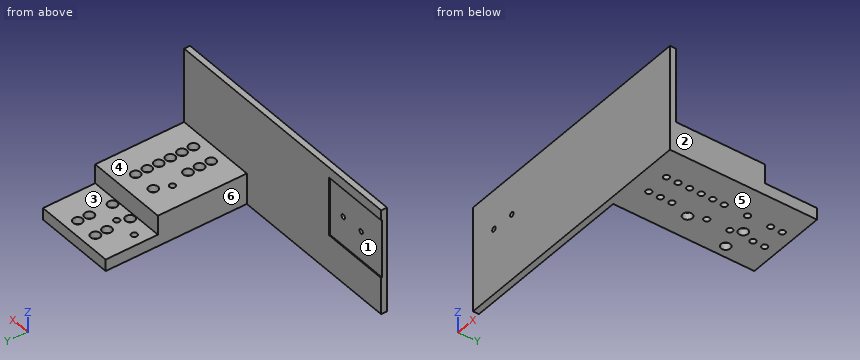
Autodesk Inventor part; units mm, degrees
ref_plane "YZ Plane" through (0, 0, 0) normal (1, 0, 0) x (0, 1, 0)
ref_plane "XZ Plane" through (0, 0, 0) normal (0, 1, 0) x (-1, 0, 0)
ref_plane "XY Plane" through (0, 0, 0) normal (0, 0, 1) x (1, 0, 0)
sketch "Sketch1" plane through (0, 0, 0) normal (0, 0, 1) x (1, 0, 0)
  line L0 (44.45, 76.2) -> (-44.45, 76.2)
  line L1 (-44.45, 76.2) -> (-44.45, -76.2)
  line L2 (-44.45, -76.2) -> (44.45, -76.2)
  line L3 (44.45, -76.2) -> (44.45, 76.2)
  line L4 (44.45, 76.2) -> (-44.45, -76.2) construction
  line L5 (-44.45, 76.2) -> (44.45, -76.2) construction
  point P0 (0, 0)
  dimension "d0" = 152.4
  dimension "d1" = 88.9
extrude "Extrusion1" add sketch "Sketch1" along normal blind 12.7
sketch "Sketch2" plane through (0, 0, 12.7) normal (0, 0, 1) x (1, 0, 0)
  line L0 (-44.45, 76.2) -> (-44.45, -76.2)
  line L1 (44.45, -76.2) -> (44.45, 76.2)
  line L2 (-44.45, -76.2) -> (44.45, -76.2)
  line L3 (44.45, -76.2) -> (44.45, 19.812)
  line L4 (44.45, 19.812) -> (-44.45, 19.812)
  line L5 (-44.45, 19.812) -> (-44.45, -76.2)
  point P0 (0, 0)
  dimension "d4" = 96.012
extrude "Extrusion2" add sketch "Sketch2" along normal blind 20.828
sketch "Sketch3" plane through (0, 0, 0) normal (0, 0, -1) x (-1, 0, 0)
  line L0 (-44.45, -76.2) -> (-44.45, 76.2)
  line L1 (44.45, -76.2) -> (-44.45, -76.2)
  point P0 (0, 0)
  point P1 (19.05, -15.24)
  dimension "d14" = 63.5
  dimension "d15" = 60.96
hole "Hole1" at (-19.05, -15.24, 0) direction (0, 0, 1) diameter 6.35 end through all counterbore diameter 10.16 counterbore depth 7.62
sketch "Sketch4" plane through (0, 0, 0) normal (0, 0, -1) x (-1, 0, 0)
  line L0 (44.45, -76.2) -> (-44.45, -76.2)
  line L1 (-44.45, -76.2) -> (-44.45, 76.2)
  point P0 (0, 0)
  point P1 (32.1564, 35.937)
  point P2 (44.45, 19.812)
  dimension "d24" = 76.6064
  dimension "d155" = 16.125
hole "Hole2" at (-32.1564, 35.937, 0) direction (0, 0, 1) diameter 6.35 end through all counterbore diameter 10.16 counterbore depth 7.62
pattern_linear "Rectangular Pattern1" count 2 spacing 25 along (1, 0, 0) of "Hole2"
sketch "Sketch5" plane through (0, 0, 12.7) normal (0, 0, 1) x (1, 0, 0)
  line L0 (-44.45, 76.2) -> (-44.45, 19.812)
  line L1 (44.45, 76.2) -> (-44.45, 76.2)
  point P0 (0, 0)
  point P1 (-12.5, 62.9666)
  dimension "d35" = 31.95
  dimension "d36" = 13.2334
hole "Hole3" at (-12.5, 62.9666, 12.7) direction (0, 0, -1) diameter 6.35 end through all counterbore diameter 10.16 counterbore depth 7.62
pattern_linear "Rectangular Pattern2" count 2 spacing 25 along (1, 0, 0) count 2 spacing 12.5 along (0, -1, 0) of "Hole3"
sketch "Sketch6" plane through (0, 0, 12.7) normal (0, 0, 1) x (1, 0, 0)
  circle A0 centre (-12.5, 50.4666) radius 5.08
  line L0 (-44.45, 76.2) -> (-44.45, 19.812)
  point P0 (0, 0)
  point P1 (-12.5, 25.4666)
  dimension "d50" = 25
  dimension "d51" = 31.95
hole "Hole4" at (-12.5, 25.4666, 12.7) direction (0, 0, -1) diameter 6.35 end through all counterbore diameter 10.16 counterbore depth 7.62
pattern_linear "Rectangular Pattern3" count 2 spacing 25 along (1, 0, 0) of "Hole4"
sketch "Sketch7" plane through (0, 0, 33.528) normal (0, 0, 1) x (1, 0, 0)
  line L0 (-44.45, 19.812) -> (-44.45, -76.2)
  circle A0 centre (-12.5, 25.4666) radius 3.175
  point P0 (0, 0)
  point P1 (-12.5, 0.4666)
  dimension "d62" = 31.95
  dimension "d63" = 25
hole "Hole5" at (-12.5, 0.4666, 33.528) direction (0, 0, -1) diameter 6.35 end through all counterbore diameter 10.16 counterbore depth 7.62
pattern_linear "Rectangular Pattern4" count 2 spacing 25 along (1, 0, 0) of "Hole5"
sketch "Sketch8" plane through (0, 0, 33.528) normal (0, 0, 1) x (1, 0, 0)
  line L0 (-44.45, 19.812) -> (-44.45, -76.2)
  circle A0 centre (-12.5, 0.4666) radius 5.08
  point P0 (0, 0)
  point P1 (-12.5, -37.0334)
  dimension "d74" = 31.95
  dimension "d75" = 37.5
hole "Hole6" at (-12.5, -37.0334, 33.528) direction (0, 0, -1) diameter 6.35 end through all counterbore diameter 10.16 counterbore depth 7.62
pattern_linear "Rectangular Pattern5" count 2 spacing 25 along (1, 0, 0) count 3 spacing 12.5 along (0, -1, 0) of "Hole6"
sketch "Sketch9" plane through (0, 0, 33.528) normal (0, 0, 1) x (1, 0, 0)
  line L0 (44.45, -76.2) -> (44.45, 19.812)
  circle A0 centre (12.5, 0.4666) radius 5.08
  point P0 (0, 0)
  point P1 (12.5, -12.0334)
  dimension "d89" = 31.95
  dimension "d90" = 12.5
hole "Hole7" at (12.5, -12.0334, 33.528) direction (0, 0, -1) diameter 6.35 end through all counterbore diameter 10.16 counterbore depth 7.62
pattern_linear "Rectangular Pattern6" count 2 spacing 12.5 along (0, -1, 0) of "Hole7"
sketch "Sketch13" plane through (-44.45, -76.2, 0) normal (0, -1, 0) x (1, 0, 0)
  line L0 (88.9, 0) -> (0, 0)
  line L1 (88.9, 0) -> (-190.5, 0)
  line L2 (-190.5, 0) -> (-190.5, 114.3)
  line L3 (-190.5, 114.3) -> (88.9, 114.3)
  line L4 (88.9, 114.3) -> (88.9, 0)
  point P0 (44.45, 0)
  dimension "d133" = 279.4
  dimension "d134" = 114.3
extrude "Extrusion3" add sketch "Sketch13" along normal blind 6.35
sketch "Sketch14" plane through (-44.45, -76.2, 0) normal (0, 1, 0) x (1, 0, 0)
  line L0 (88.9, 0) -> (88.9, -114.3)
  line L1 (-190.5, 0) -> (0, 0)
  point P0 (44.45, 0)
  point P1 (-135.4328, -71.628)
  dimension "d144" = 224.3328
  dimension "d145" = 71.628
hole "Hole11" at (-179.8828, -76.2, 71.628) direction (0, -1, 0) diameter 4.9784 end through all
pattern_linear "Rectangular Pattern10" count 2 spacing 25.4 along (-1, 0, 0) of "Hole11"
sketch "Sketch15" plane through (-44.45, -76.2, 0) normal (0, 1, 0) x (1, 0, 0)
  line L0 (-116.3828, -39.878) -> (-192.5828, -39.878)
  line L1 (-192.5828, -39.878) -> (-192.5828, -103.378)
  line L2 (-192.5828, -103.378) -> (-116.3828, -103.378)
  line L3 (-116.3828, -103.378) -> (-116.3828, -39.878)
  circle A0 centre (-135.4328, -71.628) radius 2.4892
  point P0 (44.45, 0)
  dimension "d149" = 63.5
  dimension "d150" = 76.2
  dimension "d151" = 19.05
  dimension "d152" = 31.75
extrude "Extrusion4" cut sketch "Sketch15" against normal blind 1.0414
properties part number "Baseplate as 1 V3"
Geometry: final body of the model. Coordinates: model frame, mm. Face numbers are marked on the shaded views. A direction names the side the tool comes from. Give positions to 0.01 mm unless a question says otherwise; leave off trailing zeros. Write each loop counter-clockwise with the first axis right and the second up, starting at its lowest first coordinate (ties: lowest second). Pieces come first, ordered by that corner, then holes.
1. Section query A-A, the plane x = 12.5. Count the separate pieces of the cut face and the enclosed holes in it, then the cut area to 3 significant figures.
2. Line query: probe 1 along Y at (x, z) = (-12, 29); probe 2 along X at (y, z) = (36, 5); probe 3 along Y at (x, z) = (-19.05, 21.5) (3 decimals). Output: solid intervals per line, ascending.
3. Reachability of the marked faces 4, 5 and 6 from +Z, -Z, +X, -X, +Y, -Y: full face, straight path, thin tool, end or side. Return the list, or none.
4. Section query C-C, the plane x = -97.5. Return loops of the section in (y, z).
5. Draft query along Z for the marked faces 1, 2 and 3. Return one class per face: released by +Z, released by -Z, zero draft, split by the parting line, or undercut.
6. Pin query (flat end, axial travel): P1, Ø5, axis at x = 12.5, y = -38, coming from the +Z side; P2, Ø5, axis at x = -109.5, z = 24, coming from the +Y side; P3, Ø16.5, axis at x = -32.16, y = 35.94, coming from the -Z side; P4, Ø8, axis at x = -12.5, y = 25.47, coming from the +Z side. Return the tip coordinate at first contact, or that it passes through.
7. Section query B-B, the plane z = 80. Return loops of the section in (x, y).
Computed:
1. separate pieces: 10
1. enclosed holes: 0
1. area: 2,880 mm2
2. probe 1: y = -82.55 to -67.09, -56.98 to -54.59, -44.48 to -42.09, -31.98 to -4.59, 5.52 to 19.81
2. probe 2: x = -44.45 to -37.24, -27.08 to -12.24, -2.08 to 44.45
2. probe 3: y = -82.55 to -18.415, -12.065 to 19.812
3. face 4: +Z, +X, -X, +Y
3. face 5: -Z, +X, -X, +Y, -Y
3. face 6: +Z, -Z, -X, +Y
4. outline: (-82.55, 0) - (-76.2, 0) - (-76.2, 114.3) - (-82.55, 114.3) - close
5. face 1: undercut
5. face 2: zero draft
5. face 3: released by +Z
6. P1: stops at z = 25.91
6. P2: stops at y = -76.2
6. P3: stops at z = 0
6. P4: stops at z = 5.08
7. outline: (-234.95, -82.55) - (44.45, -82.55) - (44.45, -76.2) - (-160.83, -76.2) - (-160.83, -77.24) - (-234.95, -77.24) - close
